Can you work these out from the drawing? Everything is in mm from the part's minimum corner. A direction names the side the tool comes from. Coordinates: 2 decimals unless noted, no trailing zeros. Order: outer loops, then holes, each group sorted by start corner. A loop starts at its lowest first (then second) coordinate and runs counter-clockwise, first axis right, second up. Notation, with made-up numbers: (59, -39.75) -> (118, -39.75) arc R31 ccw to (118, -2.75) -> close; hole circle Ø5 at (48, 54). An arc over 180 degrees is marked (long way). Put each result on its own line as item: value. Start each with the question number.
Q1. Will these pins go through, and if not, where does the flat tip stop? pin 1 (4 mm diameter, centred on x = 9, z = 5, fed in from +Y); pin 2 (2 mm diameter, centred on y = 1.5, z = 6.5, fed in from +X); pin 3 (4.5 mm diameter, centred on y = 14, z = 11, fed in from -X).
Q2. We'd pull the mould along Z, two halves only. Please class the marked faces 4, 5 and 6: +Z half, -Z half, draft (parallel to the pull), parting line (faces both ways), or undercut.
Q3. If we section it at D-D (x = 7.5): Please give me the cut outline in (y, z).
Q4. If we section it at A-A (y = 18): Please give me the cut outline in (x, z).
Q5. For the marked faces 1, 2 and 3, which set-ups out of +Z, -Z, +X, -X, +Y, -Y let a thin tool reach every point of the face, with its end or its side?
Q6. If we section it at B-B (z = 15): Please give me the cut outline in (x, y), and give its area (3 significant figures).
Q7. Please list where these lines run through material, in increasing order: line 1 along Z through (x, y) = (5, 18); line 2 along Y through (x, z) = (2, 7.5); line 3 along X through (y, z) = (11.5, 15.75).
Q8. If we section it at C-C (x = 6): Please give me the cut outline in (y, z).
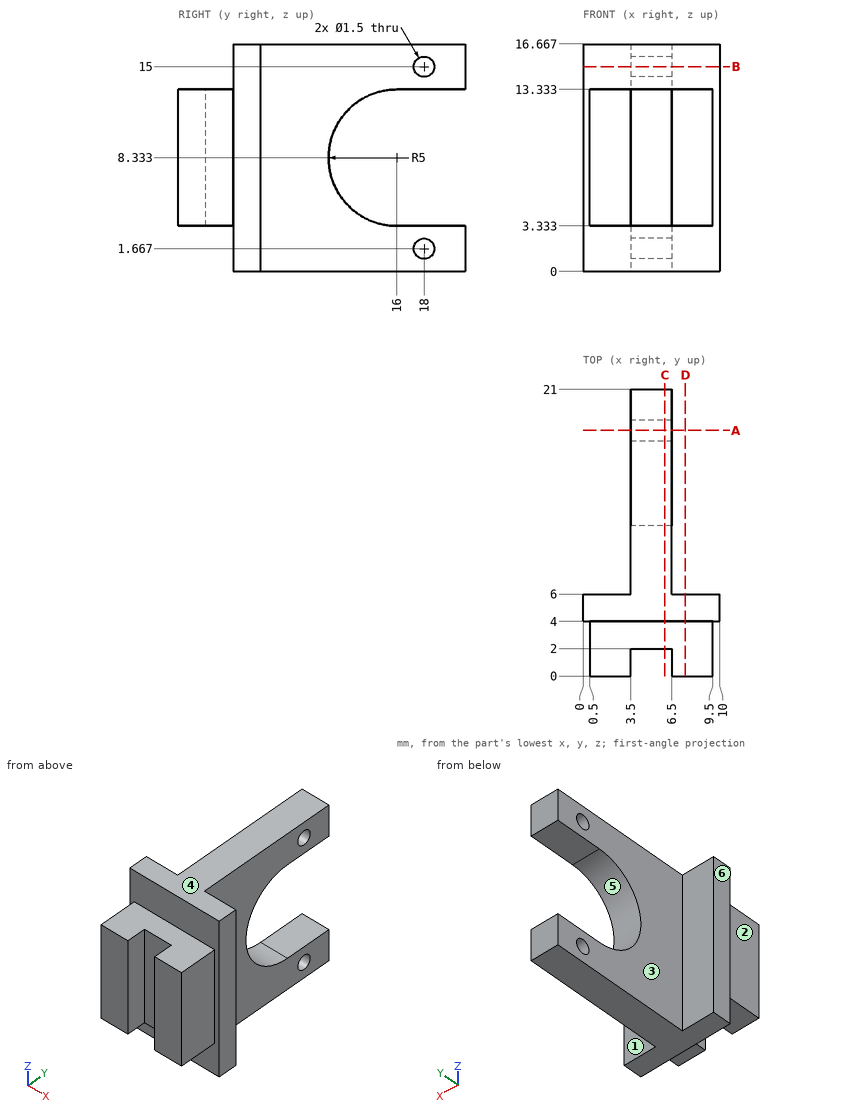
The answers:
1. pin 1: y = 6
1. pin 2: x = 9.5
1. pin 3: x = 3.5
2. face 4: +Z half
2. face 5: undercut
2. face 6: draft
3. outline: (0, 3.33) -> (4, 3.33) -> (4, 0) -> (6, 0) -> (6, 16.67) -> (4, 16.67) -> (4, 13.33) -> (0, 13.33) -> close
4. outline: (3.5, 0) -> (6.5, 0) -> (6.5, 0.92) -> (3.5, 0.92) -> close; (3.5, 2.42) -> (6.5, 2.42) -> (6.5, 3.33) -> (3.5, 3.33) -> close; (3.5, 13.33) -> (6.5, 13.33) -> (6.5, 14.25) -> (3.5, 14.25) -> close; (3.5, 15.75) -> (6.5, 15.75) -> (6.5, 16.67) -> (3.5, 16.67) -> close
5. face 1: +Z, -Z, +X, +Y
5. face 2: +Z, -Z, -X, -Y
5. face 3: +Z, -Z, -X, +Y
6. outline: (0, 4) -> (10, 4) -> (10, 6) -> (6.5, 6) -> (6.5, 17.25) -> (3.5, 17.25) -> (3.5, 6) -> (0, 6) -> close; (3.5, 18.75) -> (6.5, 18.75) -> (6.5, 21) -> (3.5, 21) -> close
6. area: 60.5 mm^2
7. line 1: 0 to 0.92, 2.42 to 3.33, 13.33 to 14.25, 15.75 to 16.67
7. line 2: 0 to 6
7. line 3: 3.5 to 6.5
8. outline: (2, 3.33) -> (4, 3.33) -> (4, 0) -> (21, 0) -> (21, 3.33) -> (16, 3.33) arc R5 cw to (16, 13.33) -> (21, 13.33) -> (21, 16.67) -> (4, 16.67) -> (4, 13.33) -> (2, 13.33) -> close; hole circle Ø1.5 at (18, 1.67); hole circle Ø1.5 at (18, 15)
